Read the model definition and answer for the solid it produces. Units are mm, in the model's axes. A direction names the side the tool comes from. Give positions to 0.01 mm unless a question says otherwise; leave off trailing zeros. Loops run counter-clockwise (first coordinate to the right, second up) from the corner with the lowest first, then second, coordinate; pieces in that order, holes last. Notation, with made-up numbers: (14, 51) - (68, 51) arc R16 cw to (68, 74) - close; hole circle Ø2 at (-30, -17). An arc over 180 degrees is marked (long way). Use a Markdown table: item, result. Add a question column.
Item 1: Each of these flat-tipped pins is pushed along its axis until it touches: P1, Ø5, axis at x = 7.5, z = 22.5, coming from the +Y side (3 decimals); P2, Ø1, axis at x = 5.5, y = 7.5, coming from the +Z side; P3, Ø3, axis at x = 3, z = 19, coming from the -Y side (3 decimals). Where does it stop, or does it pass through?
Item 2: For a pull along Y with two mould halves and no side action, classify faces 4 (the face through (5, 0, 3)), 5 (the face through (3.1, 6.58, 3.13)), 6 (the face through (4.696, 21.27, 24.495)) as +Y half, -Y half, draft (parallel to the pull), parting line (faces both ways), or undercut.
Item 3: A cutting plane is placed at C-C (y = 4.5). Determine the outline of the cut face in (x, z) (3 decimals), plus the area to 3 significant figures.
Item 4: Which of the six approach directions +Z, -Z, +X, -X, +Y, -Y give full straight-line access (tool end or side, diameter ignored) to faces 1 (the face through (3, 25, 6.35)), 2 (the face through (4.02, 24.64, 3.13)), 3 (the face through (3, 7, 6.35))?
Item 5: A cutting plane is placed at A-A (x = 5.25). Determine the outline of the cut face in (y, z) (3 decimals).
Item 6: A cutting plane is placed at D-D (z = 5.5). Give the number of separate pieces and of enclosed holes in the cut face, plus the area to 3 significant figures.
Item 7: Consider probe 1 along Y at (x, z) = (6.25, 19.05) (3 decimals); probe 2 along Y at (x, z) = (4, 1.5); probe 3 along Z at (x, y) = (1.25, 8). Determine where each line is inside the solid, lowest interval first. Write a range as [from, to].
Item 8: A cutting plane is placed at B-B (z = 19.05). Determine the outline of the cut face in (x, y) (3 decimals), plus the area to 3 significant figures.
Autodesk Inventor part; units mm, degrees
ref_plane "YZ Plane" through (0, 0, 0) normal (1, 0, 0) x (0, 1, 0)
ref_plane "XZ Plane" through (0, 0, 0) normal (0, 1, 0) x (-1, 0, 0)
ref_plane "XY Plane" through (0, 0, 0) normal (0, 0, 1) x (1, 0, 0)
sketch "Sketch1" plane through (0, 0, 0) normal (0, 0, 1) x (1, 0, 0)
  line L0 (0, 0) -> (9.525, 0)
  line L1 (9.525, 0) -> (9.525, 31.75)
  line L2 (9.525, 31.75) -> (0, 31.75)
  line L3 (0, 31.75) -> (0, 0)
  dimension "d0" = 9.525
  dimension "d1" = 31.75
extrude "Extrusion1" add sketch "Sketch1" along normal blind 25.4
sketch "Sketch2" plane through (9.525, 0, 0) normal (1, 0, 0) x (0, 0, -1)
  line L0 (-25.4, 0) -> (-25.4, 31.75)
  line L1 (-25.4, 31.75) -> (-6.35, 31.75)
  line L2 (-6.35, 31.75) -> (-6.35, 22.225)
  line L3 (-6.35, 22.225) -> (-25.4, 22.225)
  line L4 (-25.4, 22.225) -> (-25.4, 31.75)
  line L5 (0, 0) -> (-25.4, 0)
  line L6 (-25.4, 0) -> (-6.35, 0)
  line L7 (-6.35, 0) -> (-6.35, 9.525)
  line L8 (-6.35, 9.525) -> (-25.4, 9.525)
  line L9 (-25.4, 9.525) -> (-25.4, 0)
  dimension "d4" = 9.525
  dimension "d5" = 9.525
  dimension "d6" = 19.05
  dimension "d7" = 19.05
extrude "Extrusion2" cut sketch "Sketch2" against normal blind 25.4
fillet "Fillet1" radius 3.175 4 edges at (9.525, 31.75, 3.175) (0, 31.75, 3.175) (9.525, 0, 3.175) (0, 0, 3.175)
fillet "Fillet2" radius 3.175 2 edges at (4.7625, 9.525, 25.4) (4.7625, 22.225, 25.4)
sketch "Sketch3" plane through (9.525, 3.175, 0) normal (1, 0, 0) x (0, 0, -1)
  line L0 (-22.225, 6.35) -> (-6.35, 6.35)
  line L1 (-6.35, 19.05) -> (-22.225, 19.05)
  line L2 (0, 0) -> (0, 25.4)
  point P0 (0, -3.175)
  point P1 (-19.05, 12.7)
  dimension "d12" = 6.35
  dimension "d13" = 6.35
  dimension "d14" = 19.05
hole "Hole1" at (9.525, 15.875, 19.05) direction (-1, 0, 0) diameter 4.9276 depth 25.4 tip angle 118
sketch "Sketch4" plane through (0, 22.225, 6.35) normal (0, 0, 1) x (1, 0, 0)
  line L0 (0, 0) -> (0, 6.35)
  line L1 (9.525, 6.35) -> (9.525, 0)
  line L2 (0, -19.05) -> (0, -12.7)
  line L3 (9.525, -12.7) -> (9.525, -19.05)
  line L4 (6.35, -22.225) -> (3.175, -22.225)
  line L5 (3.175, 9.525) -> (6.35, 9.525)
  point P0 (0, -22.225)
  point P1 (4.7625, -17.4625)
  point P2 (4.7625, 4.7625)
  dimension "d22" = 4.7625
  dimension "d23" = 4.7625
  dimension "d24" = 4.7625
  dimension "d25" = 4.7625
  dimension "d26" = 4.7625
  dimension "d27" = 4.7625
  dimension "d28" = 22.225
hole "Hole2" at (4.7625, 4.7625, 6.35) at (4.7625, 26.9875, 6.35) direction (0, 0, -1) diameter 4.9276 depth 25.4 tip angle 118
equation "\"d5\" = d4"
equation "\"d7\" = d6"
properties part number "FTC Piv moount"
Geometry says:
| question | item | result |
|---|---|---|
| 1 | P1 | y = 22.225 |
| 1 | P2 | z = 6.35 |
| 1 | P3 | y = 9.525 |
| 2 | face 4 | -Y half |
| 2 | face 5 | undercut |
| 2 | face 6 | +Y half |
| 3 | outline | (0, 0) - (2.313, 0) - (2.313, 6.35) - (0, 6.35) - close; (7.212, 0) - (9.525, 0) - (9.525, 6.35) - (7.212, 6.35) - close |
| 3 | area | 29.4 mm² |
| 4 | face 1 | +Z, +X, -X, +Y |
| 4 | face 2 | +Z, -Z |
| 4 | face 3 | +Z, +X, -X, -Y |
| 5 | outline | (0, 0) - (2.347, 0) - (2.347, 6.35) - (0, 6.35) - close; (7.178, 0) - (24.572, 0) - (24.572, 6.35) - (22.225, 6.35) - (22.225, 22.225) arc R3.175 ccw to (19.05, 25.4) - (12.7, 25.4) arc R3.175 ccw to (9.525, 22.225) - (9.525, 6.35) - (7.178, 6.35) - close; (29.403, 0) - (31.75, 0) - (31.75, 6.35) - (29.403, 6.35) - close; hole circle Ø4.928 at (15.875, 19.05) |
| 6 | separate pieces | 1 |
| 6 | enclosed holes | 2 |
| 6 | area | 256 mm² |
| 7 | probe 1 | [9.525, 13.411], [18.339, 22.225] |
| 7 | probe 2 | [0, 2.42], [7.11, 24.64], [29.33, 31.75] |
| 7 | probe 3 | [0, 6.35] |
| 8 | outline | (0, 9.525) - (9.525, 9.525) - (9.525, 13.411) - (0, 13.411) - close; (0, 18.339) - (9.525, 18.339) - (9.525, 22.225) - (0, 22.225) - close |
| 8 | area | 74.0 mm² |
